Here's the drawing with two shaded views (mm, measured from the low corner). I have some questions. A direction names the side the tool comes from. Give positions to 0.01 mm unless a question says otherwise; leave off trailing zeros. Write each loop counter-clockwise with the first axis right and the second up, starting at its lowest first coordinate (ties: lowest second). Pieces come first, ordered by that corner, then holes.
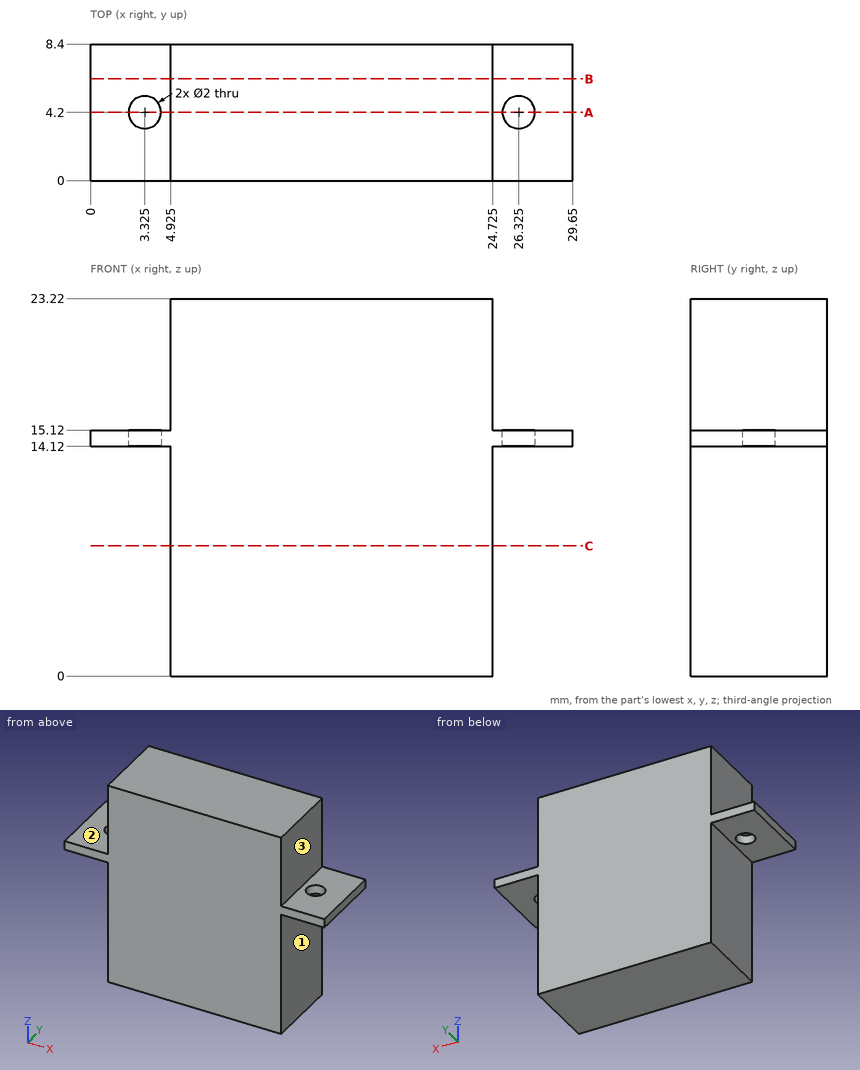
1) Suppose I cut it at A-A on y = 4.2. Write out the boundary of the cut face in (x, z) (3 decimals), plus the area to 3 significant figures.
Values follow:
outline: (0, 14.12) - (2.325, 14.12) - (2.325, 15.12) - (0, 15.12) - close; (4.325, 14.12) - (4.925, 14.12) - (4.925, 0) - (24.725, 0) - (24.725, 14.12) - (25.325, 14.12) - (25.325, 15.12) - (24.725, 15.12) - (24.725, 23.22) - (4.925, 23.22) - (4.925, 15.12) - (4.325, 15.12) - close; (27.325, 14.12) - (29.65, 14.12) - (29.65, 15.12) - (27.325, 15.12) - close
area: 466 mm2
2) Please list where these lines run through material, in increasing order: L1, parallel to X at y = 4.25, z = 9.75 (3 decimals); L2, parallel to Z at x = 2.5, y = 1.75.
Values follow:
L1: x = 4.925 to 24.725
L2: z = 14.12 to 15.12
3) For pin 1 Ø2 at (x, z) = (22, 11) entering from -Y; pin 2 Ø4 at (x, y) = (28, 5.5) entering from -Z; pin 3 Ø3 at (y, z) = (2.5, 9) entering from +X (3 decimals); pin 4 Ø2.5 at (x, y) = (2, 5) entering from +Z, each with a flat end and sliding along its axis, tell me the tip position at first contact or that it passes through.
Values follow:
pin 1: stops at y = 0
pin 2: stops at z = 14.12
pin 3: stops at x = 24.725
pin 4: stops at z = 15.12
4) For the marked faces 1, 2 and 3, which set-ups out of +Z, -Z, +X, -X, +Y, -Y let a thin tool reach every point of the face, with its end or its side?
Values follow:
face 1: -Z, +X, +Y, -Y
face 2: +Z, -X, +Y, -Y
face 3: +Z, +X, +Y, -Y
5) Suppose I cut it at C-C on z = 8. Write out the boundary of the cut face in (x, y) (3 decimals), plus the area to 3 significant figures.
Values follow:
outline: (4.925, 0) - (24.725, 0) - (24.725, 8.4) - (4.925, 8.4) - close
area: 166 mm2
6) Suppose I cut it at B-B on y = 6.25. Write out the boundary of the cut face in (x, z) (3 decimals), plus the area to 3 significant figures.
Values follow:
outline: (0, 14.12) - (4.925, 14.12) - (4.925, 0) - (24.725, 0) - (24.725, 14.12) - (29.65, 14.12) - (29.65, 15.12) - (24.725, 15.12) - (24.725, 23.22) - (4.925, 23.22) - (4.925, 15.12) - (0, 15.12) - close
area: 470 mm2
